Read the model definition and answer for the solid it produces. Units are mm, in the model's axes. Face numbers are marked on the shaded views. A direction names the side the tool comes from. Round coordinates to 2 decimals unless told otherwise and drop trailing zeros. Write each loop counter-clockwise with the first axis right and the second up, starting at its lowest first coordinate (ties: lowest second). Pieces come first, ordered by that corner, then holes.
from build123d import *

# Parameters (mm, degrees)
F0_W         = 3
F0_H         = 15
F1_DEPTH     = 5
F2_DEPTH     = 16
F3_T1_DEPTH  = 3
F3_T6_DEPTH  = 23
F3_T12_DEPTH = 13
F3_T17_DEPTH = 23
F3_T20_DEPTH = 12.2409987036
F4_R         = 2.6
F5_DEPTH     = 40.0010001


# Not quite as in the source:
# - a fillet or chamfer that OpenCascade refuses, or shapes differently, is made with other operations: its cross-section is extruded or revolved along the edge and cut away or added


with BuildPart() as f1:
    # F0 (on Top) → F1 (new body)
    with BuildSketch(Plane.XY):
        with BuildLine():
            Line((-34.3, 0), (-37, 0))
            Line((-37, 0), (-37, -15))
            Line((-37, -15), (-40, -15))
            Line((-40, -15), (-10, -40))
            Line((-10, -40), (0, -40))
            Line((0, -40), (0, -32.5))
            ThreePointArc((0, -32.5), (-12.5, -20), (0, -7.5))
            Line((0, -7.5), (0, 0))
            Line((0, 0), (-31.3, 0))
            Line((-31.3, 0), (-31.3, -15))
            Line((-31.3, -15), (-34.3, -15))
            Line((-34.3, -15), (-34.3, 0))
        make_face()
        with Locations((-32.8, -7.5)):
            Rectangle(F0_W, F0_H)
        with Locations((-38.5, -7.5)):
            Rectangle(F0_W, F0_H)
    extrude(amount=-F1_DEPTH)

    # F0 (on Top) → F2 (join)
    with BuildSketch(Plane.XY):
        with Locations((-32.8, -7.5)):
            Rectangle(F0_W, F0_H)
        with Locations((-38.5, -7.5)):
            Rectangle(F0_W, F0_H)
    extrude(amount=F2_DEPTH)

    # F3: fillet of radius 4 on 3 edges, made by hand

    # F3_s2 → F3_t1 (join)
    with BuildSketch(Plane.YZ.offset(-34.3)):
        with BuildLine():
            add(Edge.make_bspline(
                [(-15, 4), (-15, 0), (-19, 0)],
                knots=[0, 0, 0, 1, 1, 1], degree=2, weights=[1, 1, 1]))
            Line((-19, 0), (-15, 0))
            Line((-15, 0), (-15, 4))
        make_face()
    extrude(amount=F3_T1_DEPTH)


with BuildPart() as f3_tool4:
    # F3_s5 → F3_t6 (new body)
    with BuildSketch(Plane.YZ.offset(-44.3)):
        with BuildLine():
            add(Edge.make_bspline(
                [(-15, 4), (-15, 0), (-19, 0)],
                knots=[0, 0, 0, 1, 1, 1], degree=2, weights=[1, 1, 1]))
            Line((-19, 0), (-15, 0))
            Line((-15, 0), (-15, 4))
        make_face()
    extrude(amount=F3_T6_DEPTH)

    split(bisect_by=Plane(origin=(-23.7704918033, -28.5245901639, 0), x_dir=(0, 0, 1), z_dir=(0.6401843997, 0.7682212796, 0)), keep=Keep.TOP)

    split(bisect_by=Plane.YZ.offset(-37), keep=Keep.BOTTOM)


with BuildPart() as f1_1:
    add(f1.part)

    # F3_t3: union F3_tool4
    add(f3_tool4.part)


with BuildPart() as f3_tool10:
    # F3_s11 → F3_t12 (new body)
    with BuildSketch(Plane.YZ.offset(-50)):
        with BuildLine():
            add(Edge.make_bspline(
                [(-15, 4), (-15, 0), (-19, 0)],
                knots=[0, 0, 0, 1, 1, 1], degree=2, weights=[1, 1, 1]))
            Line((-19, 0), (-15, 0))
            Line((-15, 0), (-15, 4))
        make_face()
    extrude(amount=F3_T12_DEPTH)

    split(bisect_by=Plane(origin=(-23.7704918033, -28.5245901639, 0), x_dir=(0, 0, 1), z_dir=(0.6401843997, 0.7682212796, 0)), keep=Keep.TOP)


with BuildPart() as f1_2:
    add(f1_1.part)

    # F3_t9: union F3_tool10
    add(f3_tool10.part)


with BuildPart() as f3_tool15:
    # F3_s16 → F3_t17 (new body)
    with BuildSketch(Plane.YZ.offset(-50)):
        with BuildLine():
            add(Edge.make_bspline(
                [(-15, 4), (-15, 0), (-19, 0)],
                knots=[0, 0, 0, 1, 1, 1], degree=2, weights=[1, 1, 1]))
            Line((-19, 0), (-15, 0))
            Line((-15, 0), (-15, 4))
        make_face()
    extrude(amount=F3_T17_DEPTH)

    split(bisect_by=Plane.YZ.offset(-31.3), keep=Keep.BOTTOM)

    split(bisect_by=Plane.YZ.offset(-34.3), keep=Keep.TOP)


with BuildPart() as f1_3:
    add(f1_2.part)

    # F3_t14: union F3_tool15
    add(f3_tool15.part)

    # F3_s21 → F3_t20 (cut)
    with BuildSketch(Plane.XY.offset(-8.6204993518)):
        with BuildLine():
            add(Edge.make_bspline(
                [(-11.1125378579, -39.0728851184), (-10, -40), (-8.5518002593, -40)],
                knots=[0, 0, 0, 1, 1, 1], degree=2, weights=[1, 1, 1]))
            Line((-8.5518002593, -40), (-10, -40))
            Line((-10, -40), (-11.1125378579, -39.0728851184))
        make_face()
    extrude(amount=F3_T20_DEPTH, mode=Mode.SUBTRACT)

    # F4 (on face) → F5 (cut, through all)
    with BuildSketch(Plane(origin=(-40, 0, 0), x_dir=(0, -1, 0), z_dir=(-1, 0, 0))):
        with Locations((7.5, 8.4)):
            Circle(F4_R)
    extrude(amount=-F5_DEPTH, mode=Mode.SUBTRACT)

    # F6: F1 across plane


with BuildPart() as f1_4:
    add(f1_3.part)
    add(f1_3.part.mirror(Plane.YZ))


solid = f1_4.part
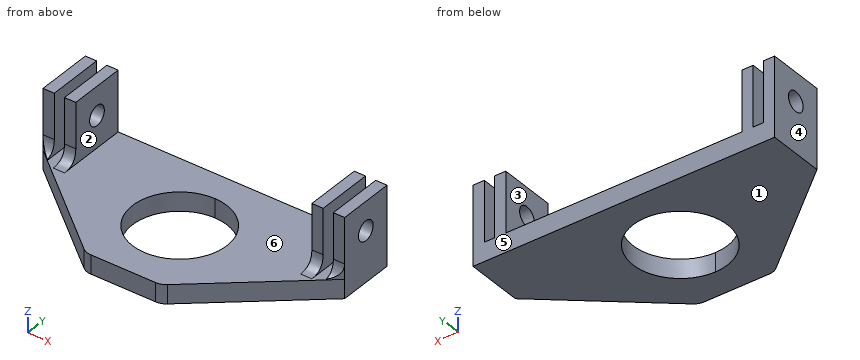
Q1. Section C-C (z = 8.4) is taken. State how many separate pieces and enclosed holes the cut face has, then the cut area to 3 significant figures.
Verdict:
separate pieces: 8
enclosed holes: 0
area: 118 mm2
Q2. Section A-A (z = 12.5) is taken. Determine the outline of the cut face in (x, y).
Verdict:
outline: (-40, -15) - (-37, -15) - (-37, 0) - (-40, 0) - close; (-34.3, -15) - (-31.3, -15) - (-31.3, 0) - (-34.3, 0) - close; (31.3, -15) - (34.3, -15) - (34.3, 0) - (31.3, 0) - close; (37, -15) - (40, -15) - (40, 0) - (37, 0) - close
Q3. Section B-B (y = -20) is taken. Determine the outline of the cut face in (x, z).
Verdict:
outline: (-34, -5) - (-12.5, -5) - (-12.5, 0) - (-34, 0) - close; (12.5, -5) - (34, -5) - (34, 0) - (12.5, 0) - close
Q4. Flat-ended cylindrical pins translate along their axes: pin 1 Ø0.9 at (x, z) = (-38, 7) entering from -Y; pin 2 Ø12 at (x, z) = (18, 0.5) entering from -Y; pin 3 Ø5 at (x, y) = (-26.5, -17) entering from +Z. Find the tip coordinate at first contact, or state that the pin passes through.
Verdict:
pin 1: stops at y = -15
pin 2: stops at y = -38.32
pin 3: stops at z = 0
Q5. Straight lines are drawn through the part: probe 1 along X at (y, z) = (-13, 10.75); probe 2 along Z at (x, y) = (38.1, -7.5); probe 3 along Z at (x, y) = (12.5, -13). For each, find the intervals that lie inside material, in ascending order.
Verdict:
probe 1: x = -40 to -37, -34.3 to -31.3, 31.3 to 34.3, 37 to 40
probe 2: z = -5 to 5.8, 11 to 16
probe 3: z = -5 to 0
Q6. Determine the mould class of the marked faces 3, 4, 5 and 6 for opening direction X: pulls with the +X half, pulls with the -X half, needs draft (parallel to the pull), parting line crosses it, or undercut.
Verdict:
face 3: undercut
face 4: pulls with the -X half
face 5: needs draft
face 6: undercut
Q7. Which of the six approach directions +Z, -Z, +X, -X, +Y, -Y give full straight-line access (tool end or side, diameter ignored) to the marked faces 1 and 2?
Verdict:
face 1: -Z, +X, -X, +Y, -Y
face 2: +Z, +Y, -Y
Q8. Section D-D (x = 7) is taken. Determine the outline of the cut face in (y, z), then the cut area to 3 significant figures.
Verdict:
outline: (-40, -5) - (-30.36, -5) - (-30.36, 0) - (-40, 0) - close; (-9.64, -5) - (0, -5) - (0, 0) - (-9.64, 0) - close
area: 96.4 mm2
